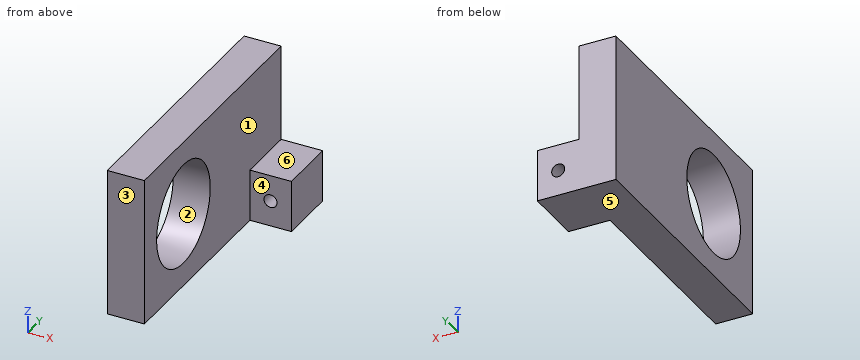
```python
from build123d import *

# Parameters (mm, degrees)
SKETCH1_W           = 6.35
SKETCH1_H           = 44.45
BOSS_EXTRUDE1_DEPTH = 25.4
SKETCH2_W           = 8.89
SKETCH2_H           = 10.16
BOSS_EXTRUDE2_DEPTH = 7.112
SKETCH4_R           = 6.441586538
CUT_EXTRUDE1_DEPTH  = 6.35
CUT_EXTRUDE2_REACH  = 41.953
SKETCH3_R           = 8.70585
SKETCH5_R           = 1.1176
SKETCH5_R_2         = 0.9906
CUT_EXTRUDE3_DEPTH  = 10.16


with BuildPart() as part:
    # Sketch1 → Boss-Extrude1 (new body)
    with BuildSketch(Plane.XY.offset(-3.193523187)):
        with Locations((-5.550476906, -10.21740419)):
            Rectangle(SKETCH1_W, SKETCH1_H)
    extrude(amount=BOSS_EXTRUDE1_DEPTH)

    # Sketch2 → Boss-Extrude2 (add)
    with BuildSketch(Plane(origin=(-2.375476906, 0, 0), x_dir=(0, 0, -1), z_dir=(1, 0, 0))):
        with Locations((-1.251476813, 6.92759581)):
            Rectangle(SKETCH2_W, SKETCH2_H)
    extrude(amount=BOSS_EXTRUDE2_DEPTH)

    # Sketch4 → Cut-Extrude1 (cut)
    with BuildSketch(Plane(origin=(-2.375476906, 0, 0), x_dir=(0, 0, -1), z_dir=(1, 0, 0))):
        with Locations(Location((-9.506476813, -19.74240419, 0), (0, 0, 90))):
            Circle(SKETCH4_R)
    extrude(amount=-CUT_EXTRUDE1_DEPTH, mode=Mode.SUBTRACT)

    # Sketch3 → Cut-Extrude2 (cut, up to next)
    with BuildSketch(Plane(origin=(-2.375476906, 0, 0), x_dir=(0, 0, -1), z_dir=(1, 0, 0)), mode=Mode.PRIVATE) as cut_extrude2_sk1:
        with Locations(Location((-9.506476813, -19.74240419, 0), (0, 0, 90))):
            Circle(SKETCH3_R)
    cut_extrude2_tool1 = extrude(cut_extrude2_sk1.sketch, amount=-CUT_EXTRUDE2_REACH, mode=Mode.PRIVATE) & part.part
    add(cut_extrude2_tool1.solids().sort_by_distance((-2.375477, -19.742404, 9.506477))[0], mode=Mode.SUBTRACT)

    # Sketch5 → Cut-Extrude3 (cut)
    with BuildSketch(Plane(origin=(0, 12.00759581, 0), x_dir=(1, 0, 0), z_dir=(0, 1, 0))):
        with Locations(Location((1.155123094, -1.192963507, 0), (0, 0, 270))):
            Circle(SKETCH5_R)
        with Locations((1.155123094, -1.192963507)):
            Circle(SKETCH5_R_2, mode=Mode.SUBTRACT)
        with Locations((1.155123094, -1.192963507)):
            Circle(SKETCH5_R_2)
    extrude(amount=-CUT_EXTRUDE3_DEPTH, mode=Mode.SUBTRACT)


solid = part.part
```
Verification items for the finished model (mm, model axes). Face numbers are marked on the shaded views. A direction names the side the tool comes from. Coordinates: 2 decimals unless noted, no trailing zeros. Loops run counter-clockwise (first coordinate to the right, second up) from the corner with the lowest first, then second, coordinate; pieces in that order, holes last. Notation, with made-up numbers: (-12.5, -21) -> (29.5, -21) arc R14 cw to (29.5, -14) -> close; hole circle Ø2 at (84, -2.5). An arc over 180 degrees is marked (long way). Answer in a Markdown table with one row per item. Add a question column.
1. Section check A-A, the plane z = 6.5. Enter the section's corners in (x, y).
2. Section check B-B, the plane y = -21.5. Enter the section's corners in (x, z).
3. Access from +Z, -Z, +X, -X, +Y, -Y to the whole of each face (thin tool, end or side, straight path). Record for the marked faces 4, 5 and 6.
4. Depth check by flat-ended pin: P1, Ø2, axis at x = -0.5, z = 1, coming from the -Y side; P2, Ø3.5, axis at x = 0.5, y = 6, coming from the +Z side; P3, Ø1.5, axis at y = -27.5, z = 18.5, coming from the +X side. Enter the tip coordinate at first touch or a pass-through.
5. Draft check along Y on the marked faces 1, 2 and 3. Enter one of: +Y half, -Y half, draft (parallel to the pull), parting line (faces both ways), or undercut.
6. Material ranges on probe 1 along Z at (x, y) = (1.25, 3); probe 2 along X at (y, z) = (0, 7.75); probe 3 along Z at (x, y) = (-1.25, 8.5), recorded low to high. Write a range as [from, to].
7. Section check D-D, the plane z = -1. Enter the section's corners in (x, y).
8. Section check C-C, the plane x = -3.5. Enter the section's corners in (y, z).
Derived:
| question | item | result |
|---|---|---|
| 1 | outline | (-8.73, -32.44) -> (-2.38, -32.44) -> (-2.38, -27.91) -> (-8.73, -27.91) -> close; (-8.73, -11.57) -> (-2.38, -11.57) -> (-2.38, 12.01) -> (-8.73, 12.01) -> close |
| 2 | outline | (-8.73, -3.19) -> (-2.38, -3.19) -> (-2.38, 0.98) -> (-8.73, 0.98) -> close; (-8.73, 18.03) -> (-2.38, 18.03) -> (-2.38, 22.21) -> (-8.73, 22.21) -> close |
| 3 | face 4 | +Z, -Z, +X, -Y |
| 3 | face 5 | -Z, +X, -X, +Y, -Y |
| 3 | face 6 | +Z, +X, +Y, -Y |
| 4 | P1 | stops at y = 1.85 |
| 4 | P2 | stops at z = 5.7 |
| 4 | P3 | stops at x = -2.38 |
| 5 | face 1 | draft |
| 5 | face 2 | undercut |
| 5 | face 3 | -Y half |
| 6 | probe 1 | z = [-3.19, 0.08], [2.31, 5.7] |
| 6 | probe 2 | x = [-8.73, -2.38] |
| 6 | probe 3 | z = [-3.19, 5.7] |
| 7 | outline | (-8.73, -32.44) -> (-2.38, -32.44) -> (-2.38, 1.85) -> (4.74, 1.85) -> (4.74, 12.01) -> (-8.73, 12.01) -> close |
| 8 | outline | (-32.44, -3.19) -> (12.01, -3.19) -> (12.01, 22.21) -> (-32.44, 22.21) -> close; hole circle Ø17.41 at (-19.74, 9.51) |
